```python
from build123d import *

# Parameters (mm, degrees)
F1_DEPTH = 25.4


with BuildPart() as f1:
    # F0 (on Top) → F1 (new body)
    with BuildSketch(Plane.XY):
        with BuildLine():
            Line((50.805587, 0), (0, 0))
            Line((0, 0), (0, -12.807356))
            Line((0, -12.807356), (16.556706, -12.807356))
            Line((16.556706, -12.807356), (16.556706, -42.451348))
            Line((16.556706, -42.451348), (6.35, -42.451348))
            ThreePointArc((6.35, -42.451348), (1.859872, -44.31122), (0, -48.801348))
            Line((0, -48.801348), (0, -49.62822))
            ThreePointArc((0, -49.62822), (1.859872, -54.118348), (6.35, -55.97822))
            Line((6.35, -55.97822), (25.748219, -55.97822))
            ThreePointArc((25.748219, -55.97822), (30.238347, -54.118348), (32.098219, -49.62822))
            Line((32.098219, -49.62822), (32.098219, -42.451348))
            Line((32.098219, -42.451348), (32.098219, -12.807356))
            Line((32.098219, -12.807356), (50.805587, -12.807356))
            Line((50.805587, -12.807356), (50.805587, 0))
        make_face()
    extrude(amount=F1_DEPTH)


solid = f1.part
```
Model file for the job. Use its own axes, mm. A direction names the side the tool comes from. Round coordinates to 2 decimals unless told otherwise and drop trailing zeros. Write each loop counter-clockwise with the first axis right and the second up, starting at its lowest first coordinate (ties: lowest second). Pieces come first, ordered by that corner, then holes. Notation, with made-up numbers: M -21.75,-4 L 33.25,-4 A26 ccw 33.25,24 Z; hole C -21.75,-16 d10. An arc over 180 degrees is marked long. Put each result on its own line as item: value.
Item 1: Mould opens along Y. For faces 4 (the flat face through (26, 0, 13)), 5 (the cylindrical face through (1.91, -44.26, 12.52)), 6 (the flat face through (32.098, -31, 13)), 7 (the cylindrical face through (30.189, -54.167, 12.522)) say: +Y half, -Y half, draft (parallel to the pull), parting line (faces both ways), or undercut.
Responses:
face 4: +Y half
face 5: undercut
face 6: draft
face 7: -Y half
Item 2: Cut at D-D (x = 5). List the corners of the cut face in (y, z), and give its area (3 significant figures).
Responses:
outline: M -55.83,0 L -42.6,0 L -42.6,25.4 L -55.83,25.4 Z; M -12.81,0 L 0,0 L 0,25.4 L -12.81,25.4 Z
area: 662 mm²
Item 3: Cut at C-C (y = -22). List the corners of the cut face in (x, z), and give its area (3 significant figures).
Responses:
outline: M 16.56,0 L 32.1,0 L 32.1,25.4 L 16.56,25.4 Z
area: 395 mm²
Item 4: Cut at B-B (x = 15.5). List the corners of the cut face in (y, z), and give its area (3 significant figures).
Responses:
outline: M -55.98,0 L -42.45,0 L -42.45,25.4 L -55.98,25.4 Z; M -12.81,0 L 0,0 L 0,25.4 L -12.81,25.4 Z
area: 669 mm²
Item 5: Flat gauge pins, fed straight in: P1, Ø1.5, axis at x = 35.5, z = 4, coming from the +Y side; P2, Ø8, axis at y = -32.5, z = 10, coming from the -X side; P3, Ø1, axis at y = -37.5, z = 7, coming from the +X side; P4, Ø5.5, axis at x = 42, z = 9.5, coming from the -Y side. Where does each tip first touch, or does it go through?
Responses:
P1: y = 0
P2: x = 16.56
P3: x = 32.1
P4: y = -12.81
Item 6: Probe L1, parallel to Y at x = 13, z = 22; L2, parallel to X at y = -18, z = 8.5; L3, parallel to Y at x = 3, z = 4. List the from-to ranges inside material, lowest first. Write a range as from..to.
Responses:
L1: -55.98..-42.45, -12.81..0
L2: 16.56..32.1
L3: -55.02..-43.41, -12.81..0
Item 7: Tool access for faces 1 (the flat face through (25, -28, 0)), 2 (the flat face through (41, -12.807, 13)), 3 (the flat face through (16.557, -27, 13)): list every direction of +Z, -Z, +X, -X, +Y, -Y with a clear straight run to the whole face (end or side of a thin tool).
Responses:
face 1: -Z, +X, -X, +Y, -Y
face 2: +Z, -Z, +X, -Y
face 3: +Z, -Z, -X
Item 8: Cut at A-A (z = 10.25). List the corners of the cut face in (x, y), and give its area (3 significant figures).
Responses:
outline: M 0,-49.63 A6.35 ccw 6.35,-55.98 L 25.75,-55.98 A6.35 ccw 32.1,-49.63 L 32.1,-12.81 L 50.81,-12.81 L 50.81,0 L 0,0 L 0,-12.81 L 16.56,-12.81 L 16.56,-42.45 L 6.35,-42.45 A6.35 ccw 0,-48.8 Z
area: 1,520 mm²
